Job drawing, mm, ordinate dimensions from the low corner. One solid piece. A direction names the side the tool comes from. Give positions to 0.01 mm unless a question says otherwise; leave off trailing zeros. Order: outer loops, then holes, each group sorted by start corner. A loop starts at its lowest first (then second) coordinate and runs counter-clockwise, first axis right, second up. Notation, with made-up numbers: (3.5, 88.25) -> (35.5, 88.25) arc R24 ccw to (35.5, 99.25) -> close; hole circle Ø6 at (27, 31.25). An arc over 180 degrees is marked (long way). Write item = value, one per line. Start each with the question number.
(1) Saw through at C-C, the plane z = 7. List the corners of the cut face in (x, y) (1 decimal).
(2) Saw through at B-B, the plane z = 33.5. List the corners of the cut face in (x, y) (1 decimal).
(3) Probe line 1 along X through (y, z) = (0.6, 28.5) (1 decimal); line 2 along Z through (x, y) = (34, 0.3) (1 decimal); line 3 along Y through (x, z) = (7, 2). List the from-to ranges inside material, lowest first. Write a range as from..to.
(4) Saw through at A-A, the plane x = 56. List the corners of the cut face in (y, z) (1 decimal), then the cut area to 3 significant figures.
(5) Flat gauge pins, fed straight in: pin 1 (0.7 mm diameter, centred on y = 0.5, z = 23.5, fed in from -X); pin 2 (7 mm diameter, centred on x = 24, z = 4, fed in from -Y). Where does each tip first touch, or does it go through?
(6) Which spindle directions (+Z, -Z, +X, -X, +Y, -Y) get a long thin tool onto all of the face, cutting with end or side? Do the marked faces 1, 2 and 3. Say none if no direction does.
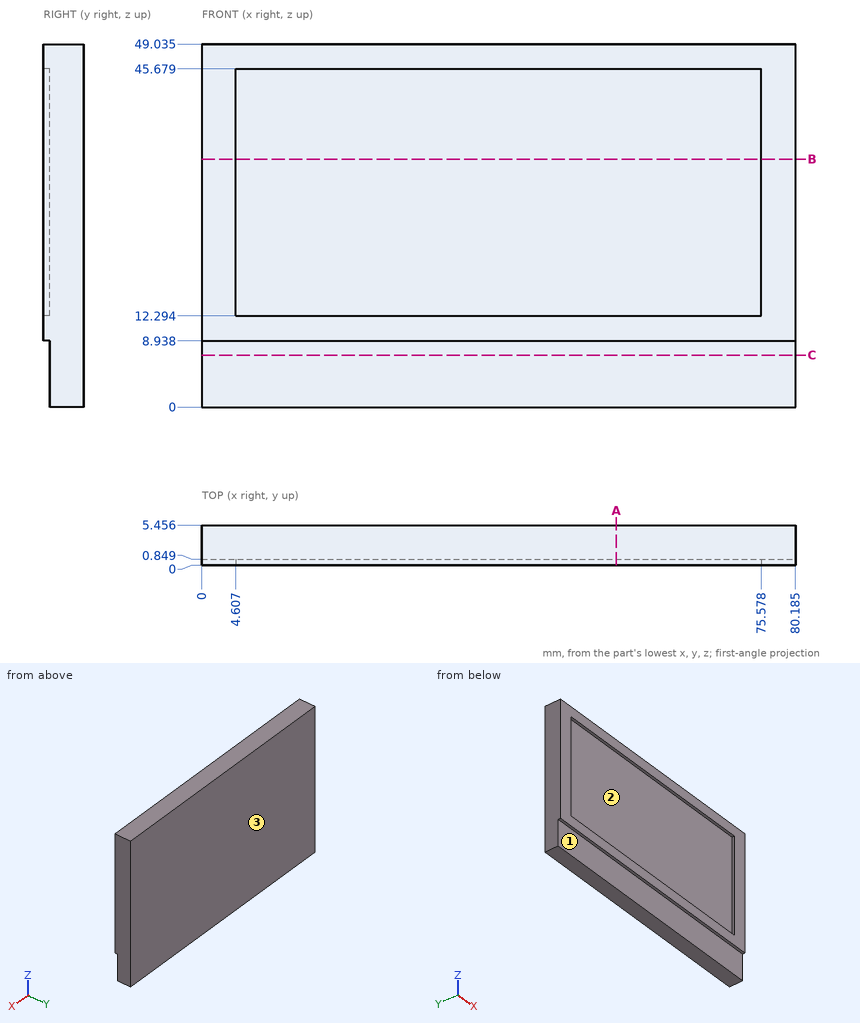
Results list:
q1.outline = (0, 0.8) -> (80.2, 0.8) -> (80.2, 5.5) -> (0, 5.5) -> close
q2.outline = (0, 0) -> (4.6, 0) -> (4.6, 0.8) -> (75.6, 0.8) -> (75.6, 0) -> (80.2, 0) -> (80.2, 5.5) -> (0, 5.5) -> close
q3.line_1 = 0..4.6, 75.6..80.2
q3.line_2 = 8.9..12.3, 45.7..49
q3.line_3 = 0.85..5.46
q4.outline = (0, 8.9) -> (0.8, 8.9) -> (0.8, 0) -> (5.5, 0) -> (5.5, 49) -> (0, 49) -> (0, 45.7) -> (0.8, 45.7) -> (0.8, 12.3) -> (0, 12.3) -> close
q4.area = 232 mm^2
q5.pin_1 = 0
q5.pin_2 = 0.85
q6.face_1 = -Z, +X, -X, -Y
q6.face_2 = -Y
q6.face_3 = +Z, -Z, +X, -X, +Y
